from build123d import *

# Parameters (mm, degrees)
F0_W     = 100
F0_H     = 100
F1_DEPTH = 50
F3_DEPTH = 142.9
F4_SIZE  = 5
F5_R     = 2


with BuildPart() as f1:
    # F0 (on Front) → F1 (new body, symmetric)
    with BuildSketch(Plane.XZ):
        Rectangle(F0_W, F0_H)
    extrude(amount=F1_DEPTH, both=True)

    # F2 (on face) → F3 (cut)
    with BuildSketch(Plane.XZ.offset(50)):
        Polygon((10.815595, -33.286978), (35, 0), (10.815595, 33.286978), (-28.315595, 20.572484), (-28.315595, -20.572484), align=None)
    extrude(amount=-F3_DEPTH, mode=Mode.SUBTRACT)

    # F4
    f4_edges = [f1.edges().sort_by_distance(p)[0] for p in [
        (50, 0, 50),
        (0, 50, 50),
        (-50, 0, 50),
        (0, -50, 50),
        (50, 50, 0),
        (50, -50, 0),
        (50, 0, -50),
        (0, 50, -50),
        (0, -50, -50),
        (-50, 0, -50),
        (-50, 50, 0),
        (-50, -50, 0),
    ]]
    chamfer(f4_edges, length=F4_SIZE)

    # F5
    f5_edges = [f1.edges().sort_by_distance(p)[0] for p in [
        (22.907797, 50, -16.643489),
        (-8.75, 50, -26.929731),
        (-28.315595, 50, 0),
        (-8.75, 50, 26.929731),
        (22.907797, 50, 16.643489),
        (22.907797, -50, -16.643489),
        (22.907797, -50, 16.643489),
        (-8.75, -50, 26.929731),
        (-28.315595, -50, 0),
        (-8.75, -50, -26.929731),
    ]]
    fillet(f5_edges, radius=F5_R)

    # F6 (on Top) → F7 (revolve)
    with BuildSketch(Plane.XY):
        Polygon((-90, 0), (-50, 0), (-50, 23.094011), align=None)
    revolve(axis=Axis((-70, 0, 0), (-1, 0, 0)))


solid = f1.part
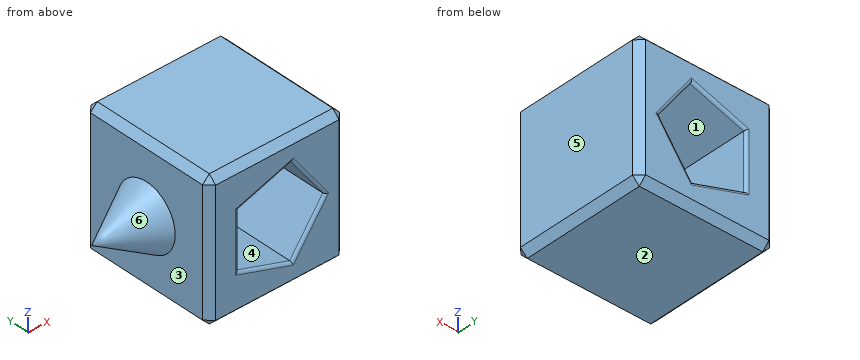
Can you work these out from the model? Positions are in its coordinate system, mm. Face numbers are marked on the shaded views. A direction names the side the tool comes from. Coordinates: 2 decimals unless noted, no trailing zeros. Write each loop counter-clockwise with the first axis right and the second up, starting at its lowest first coordinate (ties: lowest second). Pieces come first, ordered by that corner, then holes. Notation, with made-up numbers: (-0.5, 29.5) -> (30.5, 29.5) arc R20 cw to (30.5, 42.5) -> close; hole circle Ø3 at (-37.5, 74.5). An arc over 180 degrees is marked (long way). Write item = value, one per line.
(1) On a 3-axis mill with a long thin cutter (end or side, diameter ignored), from which of +Z, -Z, +X, -X, +Y, -Y can I reach the whole of each face in a straight line? I mean the marked faces 1, 2 and 3. Say none if no direction works.
Verdict:
face_1 = +Y, -Y
face_2 = -Z, +X, -X, +Y, -Y
face_3 = -X
(2) Imagine slicing it at A-A (y = 35.5). Please give me the cut outline in (x, z).
Verdict:
outline = (-50, -45) -> (-45, -50) -> (45, -50) -> (50, -45) -> (50, 45) -> (45, 50) -> (-45, 50) -> (-50, 45) -> close; hole (-28.32, -20.57) -> (10.82, -33.29) -> (35, 0) -> (10.82, 33.29) -> (-28.32, 20.57) -> close
(3) Imagine slicing it at C-C (x = -72.5). Please give me the cut outline in (y, z), and give its area (3 significant figures).
Verdict:
outline = circle Ø20.21 at (0, 0)
area = 321 mm^2
(4) If I drill on probe 1 along X at (y, z) = (-34.5, 19); probe 2 along Z at (x, y) = (20.5, -34); probe 3 along X at (y, z) = (1.5, -33.5), over which ranges is the centre line in solid material (lowest first)?
Verdict:
probe_1 = -50 to -28.32, 21.2 to 50
probe_2 = -50 to -19.96, 19.96 to 50
probe_3 = -50 to 50
(5) For pin 1 (4 mm diameter, centred on x = -50.5, y = 36.5, fed in from +Z), with a flat end and sliding along its axis, tell me the tip position at first contact or that it passes through.
Verdict:
pin_1 = 46.5
(6) Imagine slicing it at B-B (z = -38). Please give me the cut outline in (x, y).
Verdict:
outline = (-50, -45) -> (-45, -50) -> (45, -50) -> (50, -45) -> (50, 45) -> (45, 50) -> (-45, 50) -> (-50, 45) -> close
(7) Thinking about a two-plate mould opening in Z: for the marked faces 4, 5 and 6, which applies, +Z half, -Z half, draft (parallel to the pull), parting line (faces both ways), or undercut?
Verdict:
face_4 = undercut
face_5 = draft
face_6 = parting line
